Print and shaded views of the part. All mm, measured from the part's lowest x, y and z. Coordinates: 2 decimals unless noted, no trailing zeros. Order: outer loops, then holes, each group sorted by start corner. A loop starts at its lowest first (then second) coordinate and runs counter-clockwise, first axis right, second up.
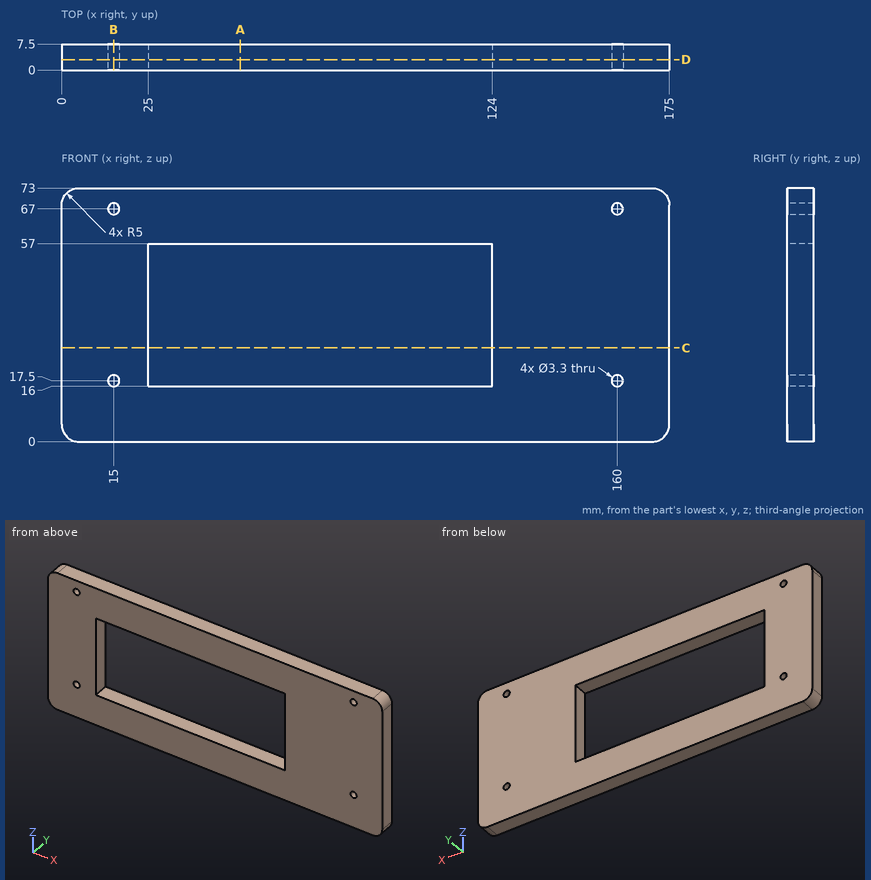
Q1. Cut at D-D, the plane y = 3. List the corners of the cut face in (x, z).
Established:
outline: (0, 5) arc R5 ccw to (5, 0) - (170, 0) arc R5 ccw to (175, 5) - (175, 68) arc R5 ccw to (170, 73) - (5, 73) arc R5 ccw to (0, 68) - close; hole circle Ø3.3 at (15, 17.5); hole circle Ø3.3 at (15, 67); hole (25, 16) - (124, 16) - (124, 57) - (25, 57) - close; hole circle Ø3.3 at (160, 17.5); hole circle Ø3.3 at (160, 67)
Q2. Cut at B-B, the plane x = 15. List the corners of the cut face in (y, z).
Established:
outline: (0, 0) - (7.5, 0) - (7.5, 15.85) - (0, 15.85) - close; (0, 19.15) - (7.5, 19.15) - (7.5, 65.35) - (0, 65.35) - close; (0, 68.65) - (7.5, 68.65) - (7.5, 73) - (0, 73) - close
Q3. Cut at A-A, the plane x = 51.5. List the corners of the cut face in (y, z).
Established:
outline: (0, 0) - (7.5, 0) - (7.5, 16) - (0, 16) - close; (0, 57) - (7.5, 57) - (7.5, 73) - (0, 73) - close
Q4. Cut at C-C, the plane z = 27. List the corners of the cut face in (x, y).
Established:
outline: (0, 0) - (25, 0) - (25, 7.5) - (0, 7.5) - close; (124, 0) - (175, 0) - (175, 7.5) - (124, 7.5) - close
Q5. Drop a flat-ended pin along its axis: P1, Ø5.5, axis at x = 160, z = 17.5, coming from the -Y side. Give the stop position or say it passes through.
Established:
P1: stops at y = 0
Q6. Probe line 1 (X direction, y = 2.75, z = 17.5); line 2 (X direction, y = 5.75, z = 67); line 3 (Z direction, x = 15, y = 4.25). List the from-to ranges inside material, lowest first.
Established:
line 1: x = 0 to 13.35, 16.65 to 25, 124 to 158.35, 161.65 to 175
line 2: x = 0 to 13.35, 16.65 to 158.35, 161.65 to 175
line 3: z = 0 to 15.85, 19.15 to 65.35, 68.65 to 73
